The model under review builds one solid part; all positions refer to its coordinate system, in mm. A direction names the side the tool comes from. Give positions to 0.01 mm unless a question says otherwise; leave off trailing zeros. Order: outer loops, then holes, each group sorted by start corner. A loop starts at its lowest first (then second) coordinate and runs counter-clockwise, first axis right, second up. Notation, with made-up numbers: (26, 31.25) -> (42, 31.25) arc R32 ccw to (42, 58.25) -> close; hole circle Ø7 at (56.5, 61.25). An arc over 180 degrees is marked (long way). Use one line per item in the form item = value.
```python
from build123d import *

# Parameters (mm, degrees)
CROQUIS1_W              = 100
CROQUIS1_H              = 100
SALIENTE_EXTRUIR1_DEPTH = 20
CROQUIS2_W              = 15
CROQUIS2_H              = 15
SALIENTE_EXTRUIR2_DEPTH = 50


with BuildPart() as part:
    # Croquis1 → Saliente-Extruir1 (new body)
    with BuildSketch(Plane(origin=(0, 0, 0), x_dir=(1, 0, 0), z_dir=(0, 1, 0))):
        Rectangle(CROQUIS1_W, CROQUIS1_H)
    extrude(amount=SALIENTE_EXTRUIR1_DEPTH)

    # Croquis2 → Saliente-Extruir2 (add)
    with BuildSketch(Plane(origin=(0, 20, 0), x_dir=(1, 0, 0), z_dir=(0, 1, 0))):
        with Locations((-42.5, -12.5)):
            Rectangle(CROQUIS2_W, CROQUIS2_H)
        with Locations((-42.5, 42.5)):
            Rectangle(CROQUIS2_W, CROQUIS2_H)
        with Locations((12.5, 42.5)):
            Rectangle(CROQUIS2_W, CROQUIS2_H)
        with Locations((12.5, -12.5)):
            Rectangle(CROQUIS2_W, CROQUIS2_H)
    extrude(amount=SALIENTE_EXTRUIR2_DEPTH)

    # Croquis4 → Revolución1 (revolve)
    with BuildSketch(Plane.XY.offset(-15)):
        with BuildLine():
            Line((-15, 105), (-15, 35))
            ThreePointArc((-15, 35), (-50, 70), (-15, 105))
        make_face()
    revolve(axis=Axis((-15, 105, -15), (0, -1, 0)))


solid = part.part
```
1. The part is to be moulded in two halves that separate along Y. For faces 1 (the face through (-44, 70, -44)), 2 (the face through (5, 39, -42)), 3 (the face through (12, 39, -35)), 4 (the face through (-43, 45, 20)), say which applies: +Y half, -Y half, draft (parallel to the pull), parting line (faces both ways), or undercut.
Values:
face_1 = +Y half
face_2 = undercut
face_3 = undercut
face_4 = draft
2. Add section A-A on y = 29. Give the boundary of the cut face in (x, z), then the cut area to 3 significant figures.
Values:
outline = (-50, -50) -> (-35, -50) -> (-35, -35) -> (-50, -35) -> close; (-50, 5) -> (-35, 5) -> (-35, 20) -> (-50, 20) -> close; (5, -50) -> (20, -50) -> (20, -35) -> (5, -35) -> close; (5, 5) -> (20, 5) -> (20, 20) -> (5, 20) -> close
area = 900 mm^2
3. For pin 1 Ø10 at (x, y) = (-10, 47) entering from +Z; pin 2 Ø12 at (x, z) = (27.5, 0.5) entering from +Y; pin 3 Ø16.5 at (x, z) = (10, 13) entering from +Y, all flat-tipped, find the tip position at first contact; note any pin that passes through.
Values:
pin_1 = 14.69
pin_2 = 20
pin_3 = 89.16
4. For L1, parallel to Z at x = -38, y = 24.5; L2, parallel to Y at x = 44.5, z = -9.5; L3, parallel to Y at x = 14, z = -43, list the stretches that pass through material, from the lowest coordinate up.
Values:
L1 = -50 to -35, 5 to 20
L2 = 0 to 20
L3 = 0 to 70
5. Add section C-C on x = 12. Give the boundary of the cut face in (y, z), then the cut area to 3 significant figures.
Values:
outline = (0, -50) -> (70, -50) -> (70, -37.27) arc R22.27 ccw to (70, 7.27) -> (70, 20) -> (20, 20) -> (20, 50) -> (0, 50) -> close; hole (20, -35) -> (60.2, -35) arc R22.27 cw to (60.2, 5) -> (20, 5) -> close
area = 5,030 mm^2
6. Add section B-B on z = 15.5. Give the boundary of the cut face in (x, y).
Values:
outline = (-50, 0) -> (50, 0) -> (50, 20) -> (20, 20) -> (20, 70) -> (5, 70) -> (5, 20) -> (-35, 20) -> (-35, 70) -> (-50, 70) -> close; circle Ø34.34 at (-15, 70)
7. Tool access review of faces 5 (the face through (-44, 70, 14)), 6 (the face through (20, 45, -42)), 7 (the face through (14, 70, 14)), 8 (the face through (-1, 19, -50)), 9 (the face through (14, 70, -44)): name each direction out of +Z, -Z, +X, -X, +Y, -Y from which nothing blocks a thin tool from reaching the whole face with its end or side.
Values:
face_5 = +Z, -X, +Y
face_6 = +Z, -Z, +X, +Y
face_7 = +Z, +X, +Y
face_8 = -Z, +X, -X, +Y, -Y
face_9 = -Z, +X, +Y
8. Add section D-D on z = -41.5. Give the boundary of the cut face in (x, y), then the cut area to 3 significant figures.
Values:
outline = (-50, 0) -> (50, 0) -> (50, 20) -> (20, 20) -> (20, 70) -> (7.86, 70) arc R22.86 ccw to (-37.86, 70) -> (-50, 70) -> close; hole (-35, 20) -> (5, 20) -> (5, 58.92) arc R22.86 cw to (-35, 58.92) -> close
area = 5,100 mm^2
